Input: part model. Units: mm. Frame: model coordinates. Face numbers are marked on the shaded views. A direction names the side the tool comes from. Coordinates: 2 decimals unless noted, no trailing zeros. Order: outer loops, then holes, each group sorted by start corner. A loop starts at its lowest first (then second) coordinate and runs counter-clockwise, first axis right, second up. Notation, with made-up numbers: M 7.5,18.5 L 17.5,18.5 A20 ccw 17.5,53.5 Z; hole C 34,4.5 d7. An arc over 180 degrees is marked long. Answer in a Markdown table with one row per item.
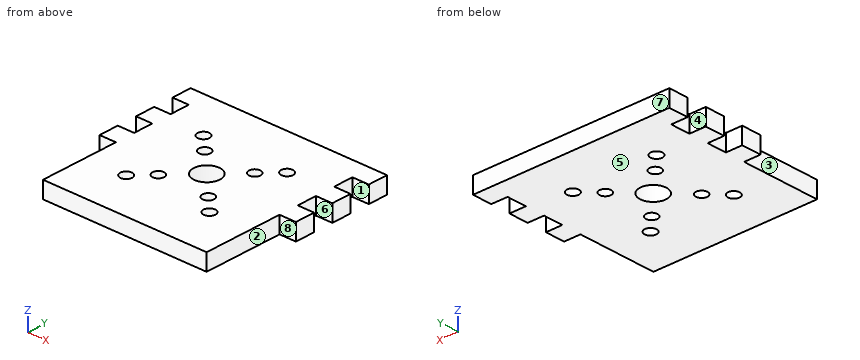
from build123d import *

# Parameters (mm, degrees)
SKETCH1_W           = 76.2
SKETCH1_H           = 76.2
BOSS_EXTRUDE1_DEPTH = 6.35
CUT_EXTRUDE1_DEPTH  = 6.35
SKETCH3_W           = 6.35
SKETCH3_H           = 38.1
CUT_EXTRUDE2_DEPTH  = 6.35
SKETCH4_W           = 6.35
SKETCH4_H           = 7.62
BOSS_EXTRUDE3_DEPTH = 6.35
SKETCH5_W           = 63.5
SKETCH5_H           = 6.35
CUT_EXTRUDE3_DEPTH  = 7.62
SKETCH6_R           = 5.08
SKETCH6_R_2         = 2.2225
SKETCH6_R_3         = 2.286
CUT_EXTRUDE4_DEPTH  = 71.769022866


with BuildPart() as part:
    # Sketch1 → Boss-Extrude1 (new body)
    with BuildSketch(Plane.XY):
        with Locations((0.21991342, -21.056709957)):
            Rectangle(SKETCH1_W, SKETCH1_H)
    extrude(amount=BOSS_EXTRUDE1_DEPTH)

    # Sketch2 → Cut-Extrude1 (cut)
    with BuildSketch(Plane.XY.offset(6.35)):
        Polygon((-37.88008658, 17.043290043), (-31.53008658, 17.043290043), (-31.53008658, 9.423290043), (-37.88008658, 9.423290043), (-37.88008658, 1.803290043), (-31.53008658, 1.803290043), (-31.53008658, -5.816709957), (-37.88008658, -5.816709957), (-37.88008658, -13.436709957), (-31.53008658, -13.436709957), (-31.53008658, -21.056709957), (-37.88008658, -21.056709957), (-46.725849744, -21.056709957), (-46.725849744, 17.043290043), align=None)
        Polygon((47.165676584, -21.056709957), (47.165676584, 17.043290043), (38.31991342, 17.043290043), (31.96991342, 17.043290043), (31.96991342, 9.423290043), (38.31991342, 9.423290043), (38.31991342, 1.803290043), (31.96991342, 1.803290043), (31.96991342, -5.816709957), (38.31991342, -5.816709957), (38.31991342, -13.436709957), (31.96991342, -13.436709957), (31.96991342, -21.056709957), (38.31991342, -21.056709957), align=None)
    extrude(amount=-CUT_EXTRUDE1_DEPTH, mode=Mode.SUBTRACT)

    # Sketch3 → Cut-Extrude2 (cut)
    with BuildSketch(Plane.XY.offset(6.35)):
        with Locations((-34.70508658, -40.106709957)):
            Rectangle(SKETCH3_W, SKETCH3_H)
        with Locations((35.14491342, -40.106709957)):
            Rectangle(SKETCH3_W, SKETCH3_H)
    extrude(amount=-CUT_EXTRUDE2_DEPTH, mode=Mode.SUBTRACT)

    # Sketch4 → Boss-Extrude3 (add)
    with BuildSketch(Plane.XY.offset(6.35)):
        with Locations((-34.70508658, -24.866709957)):
            Rectangle(SKETCH4_W, SKETCH4_H)
        with Locations((35.14491342, -24.866709957)):
            Rectangle(SKETCH4_W, SKETCH4_H)
    extrude(amount=-BOSS_EXTRUDE3_DEPTH)

    # Sketch5 → Cut-Extrude3 (cut)
    with BuildSketch(Plane(origin=(0, 17.043290043, 0), x_dir=(1, 0, 0), z_dir=(0, 1, 0))):
        with Locations((0.21991342, -3.175)):
            Rectangle(SKETCH5_W, SKETCH5_H)
    extrude(amount=-CUT_EXTRUDE3_DEPTH, mode=Mode.SUBTRACT)

    # Sketch6 → Cut-Extrude4 (cut, through all)
    with BuildSketch(Plane.XY.offset(6.35)):
        with Locations((0.21991342, -24.866709957)):
            Circle(SKETCH6_R)
        with Locations((-9.541624984, -34.62824836)):
            Circle(SKETCH6_R_2)
        with Locations((-16.005719951, -8.763829057)):
            Circle(SKETCH6_R_3)
        with Locations((-9.541419951, -15.231097531)):
            Circle(SKETCH6_R_2)
        with Locations((9.855730879, -15.231302564)):
            Circle(SKETCH6_R_2)
        with Locations((9.855525846, -34.628453393)):
            Circle(SKETCH6_R_2)
        with Locations(Location((16.445546791, -8.763829057, 0), (0, 0, 180))):
            Circle(SKETCH6_R_3)
        with Locations((16.323202085, -41.092751093)):
            Circle(SKETCH6_R_3)
        with Locations((-16.005719951, -41.092751093)):
            Circle(SKETCH6_R_3)
    extrude(amount=-CUT_EXTRUDE4_DEPTH, mode=Mode.SUBTRACT)


solid = part.part
1) Cut plane D-D, the plane y = -50.5. Output: boundary loops of the cut face in (x, z).
Resolved:
| item | result |
|---|---|
| outline | M -31.53,0 L 31.97,0 L 31.97,6.35 L -31.53,6.35 Z |
2) Cut plane A-A, the plane y = -24. Output: boundary loops of the cut face in (x, z).
Resolved:
| item | result |
|---|---|
| outline | M -37.88,0 L -4.79,0 L -4.79,6.35 L -37.88,6.35 Z; M 5.23,0 L 38.32,0 L 38.32,6.35 L 5.23,6.35 Z |
3) Mould query, pull axis Y, two halves, no side actions, for the marked faces 6, 7 and 8. Classes: +Y half, -Y half, draft (parallel to the pull), parting line (faces both ways), or undercut.
Resolved:
| item | result |
|---|---|
| face 6 | undercut |
| face 7 | +Y half |
| face 8 | -Y half |
4) Cut plane C-C, the plane z = 3.5. State how many separate pieces and enclosed holes the cut face has, and give its area (3 significant figures).
Resolved:
| item | result |
|---|---|
| separate pieces | 1 |
| enclosed holes | 9 |
| area | 4,440 mm2 |
5) Contact query for flat-ended pins moving along their axis: pin 1 (1.9 mm diameter, centred on y = -37, z = 2.5, fed in from +X); pin 2 (3.5 mm diameter, centred on x = -16.01, y = -41.09, fed in from -Z) (3 decimals); pin 3 (1.9 mm diameter, centred on x = -34, z = 3, fed in from -Y). Output: stop coordinate, or through.
Resolved:
| item | result |
|---|---|
| pin 1 | stops at x = 31.97 |
| pin 2 | passes through |
| pin 3 | stops at y = -28.68 |
6) Cut plane B-B, the plane x = 3.5. Output: boundary loops of the cut face in (y, z).
Resolved:
| item | result |
|---|---|
| outline | M -59.16,0 L -28.75,0 L -28.75,6.35 L -59.16,6.35 Z; M -20.99,0 L 9.42,0 L 9.42,6.35 L -20.99,6.35 Z |
7) Material intervals for probe 1 along Y at (x, z) = (32, 4.5); probe 2 along Y at (x, z) = (-16, 0.75); probe 3 along X at (y, z) = (-17, 5), sorted ascending.
Resolved:
| item | result |
|---|---|
| probe 1 | y = -28.68 to -21.06, -13.44 to -5.82, 1.8 to 9.42 |
| probe 2 | y = -59.16 to -43.38, -38.81 to -11.05, -6.48 to 9.42 |
| probe 3 | x = -31.53 to -10.89, -8.2 to 8.51, 11.2 to 31.97 |
8) Reachability of the marked faces 1, 2, 3, 4 and 5 from +Z, -Z, +X, -X, +Y, -Y: full face, straight path, thin tool, end or side. Return the list, or none.
Resolved:
| item | result |
|---|---|
| face 1 | +Z, -Z, +X |
| face 2 | +Z, -Z, +X, -Y |
| face 3 | +Z, -Z, -X, -Y |
| face 4 | +Z, -Z, -X |
| face 5 | -Z, +X, -X, +Y, -Y |
